The model under review builds one solid part; all positions refer to its coordinate system, in mm. A direction names the side the tool comes from. Coordinates: 2 decimals unless noted, no trailing zeros. Order: outer loops, then holes, each group sorted by start corner. A loop starts at its lowest first (then second) coordinate and runs counter-clockwise, first axis right, second up.
from build123d import *

# Parameters (mm, degrees)
BOSS_EXTRUDE1_DEPTH = 100
SKETCH2_R           = 6
CUT_EXTRUDE1_DEPTH  = 43
SKETCH4_R           = 4
CUT_EXTRUDE2_DEPTH  = 7
SKETCH6_R           = 4
CUT_EXTRUDE3_DEPTH  = 7
SKETCH7_W           = 55
SKETCH7_H           = 5
CUT_EXTRUDE4_DEPTH  = 55


with BuildPart() as part:
    # Sketch1 → Boss-Extrude1 (new body)
    with BuildSketch(Plane(origin=(0, 0, 0), x_dir=(1, 0, 0), z_dir=(0, 1, 0))):
        Polygon((0, 0), (55, 55), (0, 55), align=None)
    extrude(amount=BOSS_EXTRUDE1_DEPTH)

    # Sketch2 → Cut-Extrude1 (cut)
    with BuildSketch(Plane(origin=(50, 0, 0), x_dir=(0, 0, -1), z_dir=(1, 0, 0))):
        with Locations((17.5, 25)):
            Circle(SKETCH2_R)
        with Locations((17.5, 75)):
            Circle(SKETCH2_R)
    cut_extrude1 = extrude(amount=-CUT_EXTRUDE1_DEPTH, mode=Mode.SUBTRACT)

    # Sketch4 → Cut-Extrude2 (cut)
    with BuildSketch(Plane(origin=(7, 0, 0), x_dir=(0, 0, -1), z_dir=(1, 0, 0))):
        with Locations((17.5, 75)):
            Circle(SKETCH4_R)
        with Locations((17.5, 25)):
            Circle(SKETCH4_R)
    extrude(amount=-CUT_EXTRUDE2_DEPTH, mode=Mode.SUBTRACT)

    # Mirror6: Cut-Extrude1 across plane
    add(cut_extrude1.mirror(Plane(origin=(27.5, 0, -27.5), x_dir=(0.707106781, 0, 0.707106781), z_dir=(-0.707106781, 0, 0.707106781))), mode=Mode.SUBTRACT)

    # Sketch6 → Cut-Extrude3 (cut)
    with BuildSketch(Plane.XY.offset(-48)):
        with Locations((37.5, 75)):
            Circle(SKETCH6_R)
        with Locations((37.5, 25)):
            Circle(SKETCH6_R)
    extrude(amount=-CUT_EXTRUDE3_DEPTH, mode=Mode.SUBTRACT)

    # Sketch7 → Cut-Extrude4 (cut)
    with BuildSketch(Plane.XY):
        with Locations((27.5, 97.5)):
            Rectangle(SKETCH7_W, SKETCH7_H)
        with Locations((27.5, 2.5)):
            Rectangle(SKETCH7_W, SKETCH7_H)
    extrude(amount=-CUT_EXTRUDE4_DEPTH, mode=Mode.SUBTRACT)


solid = part.part
(1) Insertion check: pin 1 Ø6.5 at (y, z) = (25, -17.5) entering from -X; pin 2 Ø2 at (y, z) = (59, -22.5) entering from +X; pin 3 Ø13 at (y, z) = (77.5, -18) entering from +X; pin 4 Ø9.5 at (x, y) = (37.5, 75) entering from -Z. Each pin has a flat end and moves straight along its axis. Give the tip position at first contact, or say it passes through.
(2) Tool access review of faces 1 (the face through (36, 21, -48)), 2 (the face through (13.532, 26.802, -23.223)), 3 (the face through (3.549, 71.095, -16.633)): name each direction out of +Z, -Z, +X, -X, +Y, -Y from which nothing blocks a thin tool from reaching the whole face with its end or side.
(3) Consider section B-B (x = 37.5). Give the boundary of the cut face in (y, z), then the cut area to 3 significant figures.
(4) Consider section A-A (z = -17.5). Give the boundary of the cut face in (x, y).
(5) Consider section D-D (x = 9.5). Give the boundary of the cut face in (y, z), then the cut area to 3 significant figures.
(6) Consider section C-C (y = 25). Give the boundary of the cut face in (x, z), then the cut area to 3 significant figures.
(7) The part is to be moulded in two halves that separate along Z. For faces 4 (the face through (7, 21, -19)), 5 (the face through (36, 71, -48)), 6 (the face through (36.979, 28.966, -51.451)), say which applies: +Z half, -Z half, draft (parallel to the pull), parting line (faces both ways), or undercut.
(8) Wall thickness on line 1 (Y direction, x = 4, z = -17.5); line 2 (Y direction, x = 37, z = -42); line 3 (X direction, y = 75, z = -42.5): over which ranges is each line inside the solid? List them lowest first.
Findings:
1. pin 1: passes through
1. pin 2: stops at x = 23.5
1. pin 3: stops at x = 24.5
1. pin 4: stops at z = -55
2. face 1: +Z
2. face 2: +X
2. face 3: +X, -X
3. outline: (5, -55) - (21, -55) - (21, -48) - (19, -48) - (19, -37.5) - (5, -37.5) - close; (29, -55) - (71, -55) - (71, -48) - (69, -48) - (69, -37.5) - (31, -37.5) - (31, -48) - (29, -48) - close; (79, -55) - (95, -55) - (95, -37.5) - (81, -37.5) - (81, -48) - (79, -48) - close
3. area: 1,210 mm2
4. outline: (0, 5) - (17.5, 5) - (17.5, 19) - (7, 19) - (7, 21) - (0, 21) - close; (0, 29) - (7, 29) - (7, 31) - (17.5, 31) - (17.5, 69) - (7, 69) - (7, 71) - (0, 71) - close; (0, 79) - (7, 79) - (7, 81) - (17.5, 81) - (17.5, 95) - (0, 95) - close
5. outline: (5, -55) - (95, -55) - (95, -9.5) - (5, -9.5) - close; hole circle Ø12 at (25, -17.5); hole circle Ø12 at (75, -17.5)
5. area: 3,870 mm2
6. outline: (0, -55) - (33.5, -55) - (33.5, -48) - (31.5, -48) - (31.5, -31.5) - (23.5, -23.5) - (7, -23.5) - (7, -21.5) - (0, -21.5) - close; (0, -13.5) - (7, -13.5) - (7, -11.5) - (11.5, -11.5) - (0, 0) - close; (41.5, -55) - (55, -55) - (43.5, -43.5) - (43.5, -48) - (41.5, -48) - close
6. area: 1,150 mm2
7. face 4: undercut
7. face 5: +Z half
7. face 6: draft
8. line 1: y = 5 to 21, 29 to 71, 79 to 95
8. line 2: y = 5 to 19.02, 30.98 to 69.02, 80.98 to 95
8. line 3: x = 0 to 31.5
